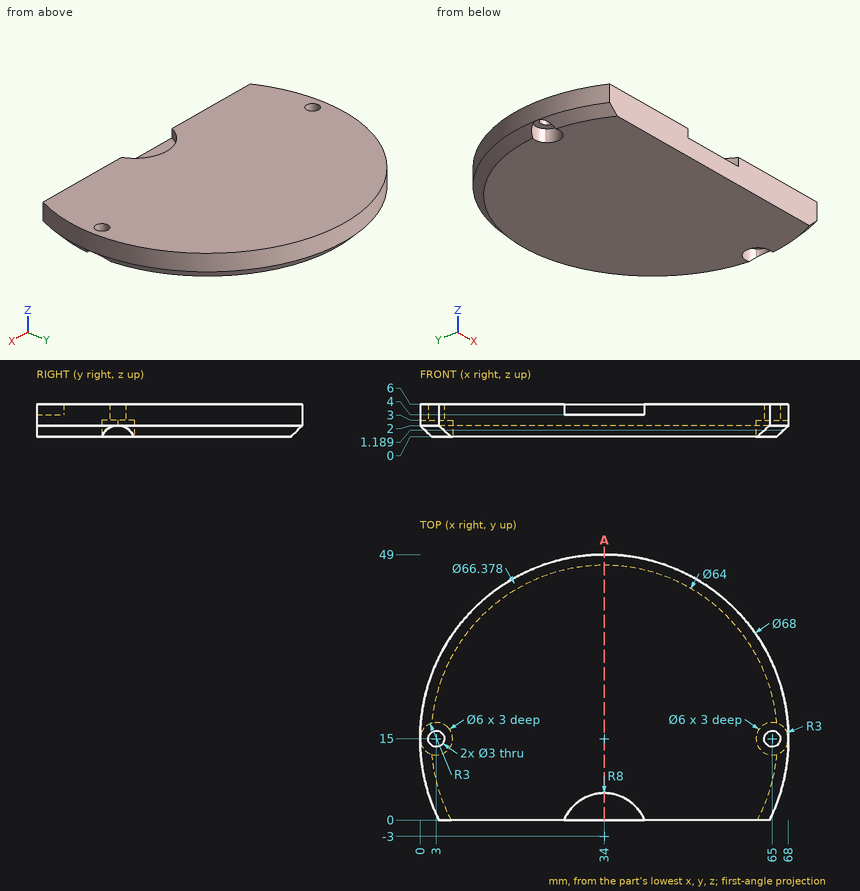
Check sheet for the drawn part. Datum: minimum x, y, z corner. Units: mm. Round coordinates to 2 decimals unless told otherwise and drop trailing zeros. Loops run counter-clockwise (first coordinate to the right, second up) from the corner with the lowest first, then second, coordinate; pieces in that order, holes last.
Item 1: Gauge pin test, flat ends, axial feed: pin 1 (2 mm diameter, centred on y = 17, z = 2, fed in from -X) (1 decimal); pin 2 (3 mm diameter, centred on x = 3.5, y = 15, fed in from -Z); pin 3 (1.8 mm diameter, centred on x = 65, y = 15.5, fed in from -Z); pin 4 (1.5 mm diameter, centred on y = 35, z = 0.5, fed in from +X) (1 decimal). Record the tip position at first contact, or that the pin passes through.
Item 2: Cross-section at A-A on x = 34. Record the boundary of the cut face in (y, z), then the cut area to 3 significant figures.
Item 3: Thickness scan on line 1 (X direction, y = 15, z = 3.85); line 2 (X direction, y = 15, z = 1.1); line 3 (Y direction, x = 65, z = 4.25) (1 decimal). Record the ranges inside material, lowest first.
Answer sheet:
1. pin 1: stops at x = 0
1. pin 2: stops at z = 3
1. pin 3: passes through
1. pin 4: stops at x = 60.7
2. outline: (0, 0) - (47, 0) - (49, 2) - (49, 6) - (5, 6) - (5, 4) - (0, 4) - close
2. area: 282 mm2
3. line 1: x = 0 to 1.5, 4.5 to 63.5, 66.5 to 68
3. line 2: x = 6 to 62
3. line 3: y = 1 to 13.5, 16.5 to 29
